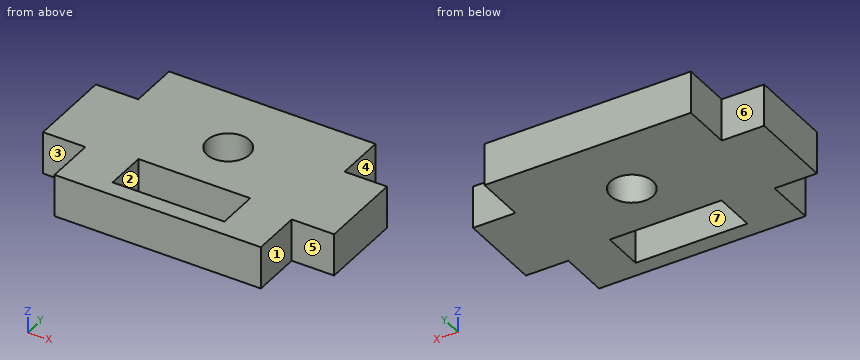
```python
from build123d import *

# Parameters (mm, degrees)
CROQUIS1_W              = 14.6
CROQUIS1_H              = 13
CROQUIS1_W_2            = 3
CROQUIS1_H_2            = 6
SALIENTE_EXTRUIR1_DEPTH = 3
CROQUIS2_R              = 1.5
CROQUIS2_W              = 7.910028885
CROQUIS2_H              = 2.9332022
CORTAR_EXTRUIR1_DEPTH   = 10


with BuildPart() as part:
    # Croquis1 → Saliente-Extruir1 (new body)
    with BuildSketch(Plane.XY):
        Rectangle(CROQUIS1_W, CROQUIS1_H)
        with Locations((-8.8, 0)):
            Rectangle(CROQUIS1_W_2, CROQUIS1_H_2)
        with Locations((8.8, 0)):
            Rectangle(CROQUIS1_W_2, CROQUIS1_H_2)
    extrude(amount=SALIENTE_EXTRUIR1_DEPTH)

    # Croquis2 → Cortar-Extruir1 (cut)
    with BuildSketch(Plane.XY.offset(3)):
        with Locations((0, 1.5)):
            Circle(CROQUIS2_R)
        with Locations((0.038370941, -3.869685697)):
            Rectangle(CROQUIS2_W, CROQUIS2_H)
    extrude(amount=-CORTAR_EXTRUIR1_DEPTH, mode=Mode.SUBTRACT)


solid = part.part
```
Geometry check sheet. Reference: the model listing, model coordinates, mm. Face numbers are marked on the shaded views. A direction names the side the tool comes from. Round coordinates to 2 decimals unless told otherwise and drop trailing zeros. Loops run counter-clockwise (first coordinate to the right, second up) from the corner with the lowest first, then second, coordinate; pieces in that order, holes last. Notation, with made-up numbers: (-22, 39) - (-5, 39) arc R21 cw to (-5, 69) - close; hole circle Ø8 at (53, 8.25). An arc over 180 degrees is marked (long way). Use a Markdown table: item, result.
Q1. Material ranges on line 1 (Y direction, x = 0, z = 1.7); line 2 (X direction, y = -2.75, z = 1.75); line 3 (Y direction, x = 2.5, z = 2.8), recorded low to high.
Solutions:
| item | result |
|---|---|
| line 1 | y = -6.5 to -5.34, -2.4 to 0, 3 to 6.5 |
| line 2 | x = -10.3 to -3.92, 3.99 to 10.3 |
| line 3 | y = -6.5 to -5.34, -2.4 to 6.5 |
Q2. Cross-section at A-A on y = 1.5. Record the cut outline in (x, z).
Solutions:
| item | result |
|---|---|
| outline | (-10.3, 0) - (-1.5, 0) - (-1.5, 3) - (-10.3, 3) - close; (1.5, 0) - (10.3, 0) - (10.3, 3) - (1.5, 3) - close |
Q3. Cross-section at D-D on x = 0. Record the cut outline in (y, z), plus the area to 3 significant figures.
Solutions:
| item | result |
|---|---|
| outline | (-6.5, 0) - (-5.34, 0) - (-5.34, 3) - (-6.5, 3) - close; (-2.4, 0) - (0, 0) - (0, 3) - (-2.4, 3) - close; (3, 0) - (6.5, 0) - (6.5, 3) - (3, 3) - close |
| area | 21.2 mm2 |
Q4. Cross-section at C-C on z = 0.2. Record the cut outline in (x, y), plus the area to 3 significant figures.
Solutions:
| item | result |
|---|---|
| outline | (-10.3, -3) - (-7.3, -3) - (-7.3, -6.5) - (7.3, -6.5) - (7.3, -3) - (10.3, -3) - (10.3, 3) - (7.3, 3) - (7.3, 6.5) - (-7.3, 6.5) - (-7.3, 3) - (-10.3, 3) - close; hole (-3.92, -5.34) - (3.99, -5.34) - (3.99, -2.4) - (-3.92, -2.4) - close; hole circle Ø3 at (0, 1.5) |
| area | 196 mm2 |
Q5. Go/stop test with flat-tipped pins: P1, Ø1.5, axis at y = -3.5, z = 1.5, coming from the -X side; P2, Ø1.5, axis at y = -4, z = 1, coming from the +X side; P3, Ø0.9, axis at x = -9.5, z = 2, coming from the -Y side. Record where each tip stops, or that it passes through.
Solutions:
| item | result |
|---|---|
| P1 | stops at x = -10.3 |
| P2 | stops at x = 7.3 |
| P3 | stops at y = -3 |
Q6. Access from +Z, -Z, +X, -X, +Y, -Y to the whole of each face (thin tool, end or side, straight path). Record for the marked faces 1, 2, 3 and 4.
Solutions:
| item | result |
|---|---|
| face 1 | +Z, -Z, +X, -Y |
| face 2 | +Z, -Z |
| face 3 | +Z, -Z, -X, -Y |
| face 4 | +Z, -Z, +X, +Y |
Q7. Draft check along Y on the marked faces 5, 6 and 7. Enter one of: released by +Y, released by -Y, zero draft, split by the parting line, or undercut.
Solutions:
| item | result |
|---|---|
| face 5 | released by -Y |
| face 6 | released by +Y |
| face 7 | undercut |
Q8. Cross-section at B-B on x = -3.25. Record the cut outline in (y, z).
Solutions:
| item | result |
|---|---|
| outline | (-6.5, 0) - (-5.34, 0) - (-5.34, 3) - (-6.5, 3) - close; (-2.4, 0) - (6.5, 0) - (6.5, 3) - (-2.4, 3) - close |
